Read the model definition and answer for the solid it produces. Units are mm, in the model's axes. A direction names the side the tool comes from. Coordinates: 2 decimals unless noted, no trailing zeros. Loops run counter-clockwise (first coordinate to the right, second up) from the corner with the lowest first, then second, coordinate; pieces in that order, holes last.
Autodesk Inventor part; units mm, degrees
ref_plane "YZ Plane" through (0, 0, 0) normal (1, 0, 0) x (0, 1, 0)
ref_plane "XZ Plane" through (0, 0, 0) normal (0, 1, 0) x (-1, 0, 0)
ref_plane "XY Plane" through (0, 0, 0) normal (0, 0, 1) x (1, 0, 0)
sketch "Sketch1" plane through (0, 0, 0) normal (0, 0, 1) x (1, 0, 0)
  line L0 (-10, -50) -> (10, -50)
  line L1 (10, -50) -> (10, 50)
  line L2 (10, 50) -> (-10, 50)
  line L3 (-10, 50) -> (-10, -50)
  line L4 (-10, -50) -> (10, 50) construction
  line L5 (10, -50) -> (-10, 50) construction
  line L6 (-8, -48) -> (8, -48)
  line L7 (8, -48) -> (8, 48)
  line L8 (8, 48) -> (-8, 48)
  line L9 (-8, 48) -> (-8, -48)
  line L10 (-8, -48) -> (8, 48) construction
  line L11 (8, -48) -> (-8, 48) construction
  point P0 (0, 0)
  dimension "d0" = 20
  dimension "d1" = 100
  dimension "d2" = 16
  dimension "d3" = 96
extrude "Extrusion1" add sketch "Sketch1" along normal blind 939
sketch "Sketch2" plane through (-10, -50, 0) normal (-1, 0, 0) x (0, 0, 1)
  circle A0 centre (199.089, 18.548) radius 16.3
  line L0 (0, 100) -> (939, 100)
  line L1 (0, 100) -> (0, 0)
  line L2 (0, 0) -> (939, 0)
  point P0 (0, 50)
  dimension "d6" = 32.6
  dimension "HoleDistanceX" = 199.089
  dimension "d11" = 18.548
extrude "Extrusion2" cut sketch "Sketch2" against normal blind 880
sketch "Sketch4" plane through (-10, -50, 0) normal (-1, 0, 0) x (0, 0, 1)
  circle A0 centre (113.659, 8.082) radius 4.5 construction
  circle A1 centre (199.089, 18.548) radius 12.25 construction
  line L0 (199.089, 18.548) -> (113.659, 8.082) construction
  line L1 (199.089, 18.548) -> (113.0203, 18.5713) construction
  circle A2 centre (113.0203, 18.5713) radius 4.5 construction
  arc A3 (113.0203, 18.5713) -> (113.659, 8.082) centre (199.089, 18.548) ccw construction
  arc A4 (113.0203, 18.5713) -> (113.659, 8.082) centre (199.089, 18.548) ccw construction
  arc A5 (108.5203, 18.5725) -> (109.1924, 7.5348) centre (199.089, 18.548) ccw
  arc A6 (117.5203, 18.5701) -> (118.1256, 8.6292) centre (199.089, 18.548) ccw
  arc A7 (117.5203, 18.5701) -> (108.5203, 18.5725) centre (113.0203, 18.5713) ccw
  arc A8 (109.1924, 7.5348) -> (118.1256, 8.6292) centre (113.659, 8.082) ccw
  line L2 (0, 0) -> (939, 0)
  line L3 (0, 100) -> (0, 0)
  point P0 (0, 50)
  dimension "d12" = 9
  dimension "d13" = 9
  dimension "d14" = 9
  dimension "d15" = 7
  dimension "d16" = 8.082
  dimension "d17" = 113.659
extrude "Extrusion3" cut sketch "Sketch4" against normal blind 3
sketch "Sketch5" plane through (-10, -50, 0) normal (-1, 0, 0) x (0, 0, 1)
  circle A0 centre (325.227, 50) radius 30
  line L0 (0, 100) -> (0, 0)
  line L1 (0, 0) -> (939, 0)
  point P0 (0, 50)
  dimension "d20" = 60
  dimension "d21" = 325.227
  dimension "d22" = 50
extrude "Extrusion4" cut sketch "Sketch5" against normal blind 3
sketch "Sketch6" plane through (-10, -50, 0) normal (-1, 0, 0) x (0, 0, 1)
  line L0 (450, 75) -> (580, 75)
  line L1 (580, 75) -> (580, 25)
  line L2 (580, 25) -> (450, 25)
  line L3 (450, 25) -> (450, 75)
  line L4 (0, 100) -> (939, 100)
  line L5 (0, 100) -> (0, 0)
  point P0 (0, 50)
  dimension "d25" = 50
  dimension "d26" = 25
  dimension "d27" = 580
  dimension "d28" = 450
extrude "Extrusion5" cut sketch "Sketch6" against normal blind 3
sketch "Sketch7" plane through (8, -48, 0) normal (-1, 0, 0) x (0, 0, 1)
  circle A0 centre (325.227, 48) radius 30
  circle A1 centre (325.227, 48) radius 9.8
  point P0 (0, 48)
  dimension "d31" = 19.6
extrude "Extrusion6" cut sketch "Sketch7" against normal through all contours A1
sketch "Sketch8" plane through (10, -50, 0) normal (1, 0, 0) x (0, 0, -1)
  circle A0 centre (-382.128, 62.7) radius 2.25
  line L0 (0, 100) -> (-939, 100)
  line L1 (0, 0) -> (0, 100)
  circle A1 centre (-382.128, 37.3) radius 2.25
  line L2 (0, 0) -> (-939, 0)
  circle A2 centre (-407.528, 62.7) radius 2.25
  circle A3 centre (-407.528, 37.3) radius 2.25
  point P0 (0, 50)
  dimension "d34" = 4.5
  dimension "d35" = 37.3
  dimension "d36" = 382.128
  dimension "d37" = 4.5
  dimension "d38" = 37.3
  dimension "d39" = 382.128
  dimension "d40" = 4.5
  dimension "d41" = 407.528
  dimension "d42" = 37.3
  dimension "d43" = 4.5
  dimension "d44" = 37.3
  dimension "d45" = 407.528
extrude "Extrusion7" cut sketch "Sketch8" against normal blind 21.1125
sketch "Sketch9" plane through (10, -50, 0) normal (1, 0, 0) x (0, 0, -1)
  circle A0 centre (-617.924, 50) radius 9.8
  line L0 (0, 100) -> (-939, 100)
  line L1 (0, 0) -> (0, 100)
  circle A1 centre (-655.408, 80) radius 2.75
  circle A2 centre (-655.408, 20) radius 2.75
  line L2 (0, 0) -> (-939, 0)
  circle A3 centre (-562, 84.5) radius 2.75
  circle A4 centre (-562, 15.5) radius 2.75
  circle A5 centre (-283.5, 20) radius 2.75
  circle A6 centre (-283.5, 80) radius 2.75
  circle A7 centre (-384.5, 84.5) radius 2.75
  circle A8 centre (-384.5, 15.5) radius 2.75
  circle A9 centre (-40, 90.5) radius 2.75
  line L3 (-40, 90.5) -> (-160, 90.5)
  line L4 (-40, 90.5) -> (80, 90.5) construction
  circle A10 centre (-160, 90.5) radius 2.75
  circle A11 centre (-100, 90.5) radius 2.75
  circle A12 centre (-903.151, 90.5) radius 2.75
  line L5 (-939, 0) -> (-939, 100)
  line L6 (-903.151, 90.5) -> (-843.151, 90.5)
  line L7 (-903.151, 90.5) -> (-843.151, 90.5) construction
  circle A13 centre (-843.151, 90.5) radius 2.75
  line L8 (-843.151, 90.5) -> (-783.151, 90.5)
  line L9 (-843.151, 90.5) -> (-783.151, 90.5) construction
  circle A14 centre (-783.151, 90.5) radius 2.75
  circle A15 centre (-637.924, 90) radius 2.75
  circle A16 centre (-597.924, 90) radius 2.75
  circle A17 centre (-627.924, 10) radius 2.75
  circle A18 centre (-597.924, 10) radius 2.75
  circle A19 centre (-345.226, 90) radius 2.75
  circle A20 centre (-305.226, 90) radius 2.75
  circle A21 centre (-315.226, 10) radius 2.75
  circle A22 centre (-345.226, 10) radius 2.75
  circle A23 centre (-682.408, 80) radius 2.75
  circle A24 centre (-682.408, 20) radius 2.75
  point P0 (0, 50)
  dimension "d48" = 19.6
  dimension "d49" = 50
  dimension "d50" = 617.924
  dimension "d53" = 5.5
  dimension "d54" = 5.5
  dimension "d55" = 20
  dimension "d56" = 20
  dimension "d57" = 655.408
  dimension "d58" = 655.408
  dimension "d60" = 5.5
  dimension "d61" = 5.5
  dimension "d62" = 15.5
  dimension "d63" = 15.5
  dimension "d64" = 562
  dimension "d65" = 562
  dimension "d66" = 5.5
  dimension "d67" = 5.5
  dimension "d68" = 283.5
  dimension "d69" = 283.5
  dimension "d70" = 20
  dimension "d71" = 20
  dimension "d72" = 5.5
  dimension "d73" = 384.5
  dimension "d74" = 15.5
  dimension "d75" = 5.5
  dimension "d76" = 384.5
  dimension "d77" = 15.5
  dimension "d92" = 5.5
  dimension "d93" = 40
  dimension "d94" = 9.5
  dimension "d95" = 120
  dimension "d96" = 180
  dimension "d97" = 5.5
  dimension "d98" = 5.5
  dimension "d99" = 60
  dimension "d100" = 5.5
  dimension "d101" = 35.849
  dimension "d102" = 9.5
  dimension "d103" = 60
  dimension "d104" = 0
  dimension "d105" = 5.5
  dimension "d106" = 60
  dimension "d107" = 0
  dimension "d108" = 5.5
  dimension "d109" = 5.5
  dimension "d110" = 301.076
  dimension "d111" = 10
  dimension "d112" = 5.5
  dimension "d113" = 10
  dimension "d114" = 40
  dimension "d115" = 5.5
  dimension "d116" = 10
  dimension "d117" = 5.5
  dimension "d118" = 10
  dimension "d119" = 40
  dimension "d120" = 30
  dimension "d121" = 5.5
  dimension "d122" = 10
  dimension "d123" = 345.226
  dimension "d124" = 5.5
  dimension "d125" = 40
  dimension "d126" = 10
  dimension "d127" = 5.5
  dimension "d128" = 80
extrude "Extrusion8" cut sketch "Sketch9" against normal blind 37.625 contours A0 | A1 | A2 | A3 | A4 | A5 | A6 | A7 | A8 | A9 | A10 | A11 L3 | L3 A11 | A12 | A14 | A13 L8 L6 | L6 L8 A13 | A15 | A16 | A17 | A18 | A19 | A20 | A21 | A22 | A23 | A24
sketch "Sketch10" plane through (-10, -50, 0) normal (-1, 0, 0) x (0, 0, 1)
  circle A0 centre (744.0619, 18.548) radius 16.3
  line L0 (0, 0) -> (939, 0)
  circle A1 centre (199.089, 18.548) radius 16.3
  circle A2 centre (617.924, 50) radius 9.8
  point P0 (0, 50)
  dimension "d78" = 32.6
  dimension "d79" = 18.548
  dimension "d83" = 126.1379
extrude "Extrusion9" cut sketch "Sketch10" against normal through all contours A0
sketch "Sketch11" plane through (-10, 50, 0) normal (0, 1, 0) x (1, 0, 0)
  circle A0 centre (10, -325.227) radius 5
  line L0 (20, 0) -> (0, 0)
  line L1 (20, 0) -> (20, -939)
  circle A1 centre (10, -617.924) radius 5
  line L2 (20, -939) -> (0, -939)
  line L3 (0, 0) -> (0, -939)
  point P0 (10, 0)
  dimension "d84" = 10
  dimension "d85" = 325.227
  dimension "d86" = 10
  dimension "d87" = 10
  dimension "d88" = 321.076
  dimension "d89" = 10
extrude "Extrusion10" cut sketch "Sketch11" against normal blind 10 contours A0 | A1
properties part number "Side Extrusion" material "Aluminum 6061"
Q1. A cutting plane is placed at A-A (x = 0). Give the vertices of the cut face in (y, z), then the cut area to 3 significant figures.
Findings below:
outline: (-50, 0) - (-48, 0) - (-48, 939) - (-50, 939) - close; (48, 0) - (50, 0) - (50, 320.23) - (48, 320.23) - close; (48, 330.23) - (50, 330.23) - (50, 612.92) - (48, 612.92) - close; (48, 622.92) - (50, 622.92) - (50, 939) - (48, 939) - close
area: 3,720 mm2
Q2. Straight lines are drawn through the part: probe 1 along Z at (x, y) = (0, 48.7); probe 2 along Y at (x, z) = (5.5, 825.5); probe 3 along X at (y, z) = (-4.5, 412). For each, find the intervals that lie inside material, in ascending order.
Findings below:
probe 1: z = 0 to 320.23, 330.23 to 612.92, 622.92 to 939
probe 2: y = -50 to -48, 48 to 50
probe 3: x = -10 to -8, 8 to 10
Q3. A cutting plane is placed at B-B (z = 142.5). Give the vertices of the cut face in (x, y).
Findings below:
outline: (-10, -50) - (10, -50) - (10, 50) - (-10, 50) - close; hole (-8, -48) - (8, -48) - (8, 48) - (-8, 48) - close
Q4. A cutting plane is placed at C-C (z = 497.5). Give the vertices of the cut face in (x, y), then the cut area to 3 significant figures.
Findings below:
outline: (-10, -50) - (10, -50) - (10, 50) - (-10, 50) - (-10, 25) - (-8, 25) - (-8, 48) - (8, 48) - (8, -48) - (-8, -48) - (-8, -25) - (-10, -25) - close
area: 364 mm2
Q5. Flat-ended cylindrical pins translate along their axes: pin 1 Ø3.5 at (y, z) = (12.7, 382.128) entering from +X; pin 2 Ø8 at (y, z) = (-20.5, 548) entering from -X. Find the tip coordinate at first contact, or state that the pin passes through.
Findings below:
pin 1: passes through
pin 2: stops at x = 8
Q6. Which of the six approach directions +Z, -Z, +X, -X, +Y, -Y give full straight-line access (tool end or side, diameter ignored) to faces 1 (the face through (-9.014, 1.319, 295.256)), 2 (the face through (8.99, -37.69, 759.12)), 3 (the face through (8, -1, 463))?
Findings below:
face 1: -X
face 2: +X, -X
face 3: +Z, -Z
Q7. Determine the mould class of faces 4 (the face through (-10, 34, 463)), 5 (the face through (-8, 33, 463)), 6 (the face through (0, -50, 463)) for opening direction X: +X half, -X half, draft (parallel to the pull), parting line (faces both ways), or undercut.
Findings below:
face 4: -X half
face 5: undercut
face 6: draft
